Read the model definition and answer for the solid it produces. Units are mm, in the model's axes. Face numbers are marked on the shaded views. A direction names the side the tool comes from. Coordinates: 2 decimals unless noted, no trailing zeros. Write each loop counter-clockwise with the first axis right and the second up, starting at its lowest first coordinate (ties: lowest second). Pieces come first, ordered by that corner, then holes.
(1) The part is cut by section A-A, the plane z = 0. State how many separate pieces and enclosed holes the cut face has, and give its area (3 significant figures).
(2) Straight lines are drawn through the part: line 1 along X through (y, z) = (71, 12); line 2 along X through (y, z) = (11.25, 0); line 3 along Y through (x, z) = (16, 0). For each, find the intervals that lie inside material, in ascending order.
(3) Given pin 1 (8 mm diameter, centred on y = 54, z = -11, fed in from +X); pin 2 (9 mm diameter, centred on x = 13.5, y = 62, fed in from +Z); pin 3 (5.5 mm diameter, centred on y = 11, z = 18.5, fed in from -X); pin 4 (8 mm diameter, centred on x = -22, y = 39.5, fed in from -Z), each flat-ended and moving along its own axis, determine where each tip first touches the part or whether it passes through.
(4) The part is cut by section C-C, the plane x = -4. Determine the outline of the cut face in (y, z), and give its area (3 significant figures).
(5) The part is cut by section D-D, the plane y = 20. Determine the outline of the cut face in (x, z).
(6) Which of the six approach directions +Z, -Z, +X, -X, +Y, -Y give full straight-line access (tool end or side, diameter ignored) to the marked faces 4, 5 and 6?
(7) The part is cut by section B-B, the plane y = 79. Determine the outline of the cut face in (x, z).
(8) Determine the mould class of the marked faces 1, 2 and 3 for opening direction Y: pulls with the +Y half, pulls with the -Y half, needs draft (parallel to the pull), parting line crosses it, or undercut.
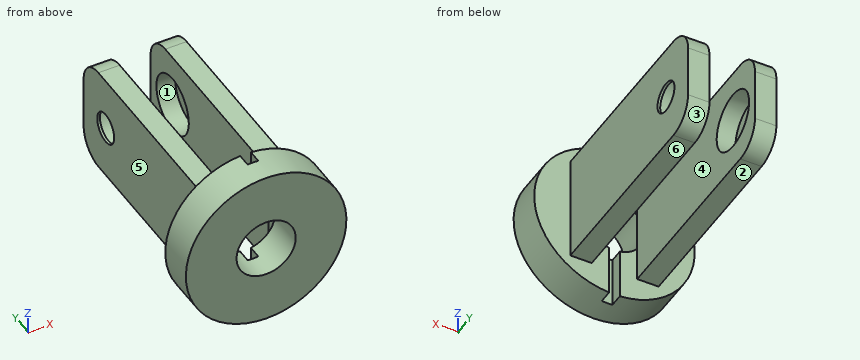
```python
from build123d import *

# Parameters (mm, degrees)
SKETCH1_R               = 30
BOSS_EXTRUDE1_DEPTH     = 14
SKETCH2_R               = 11.05
CUT_EXTRUDE1_DEPTH      = 45.676615807
SKETCH5_W               = 8
SKETCH5_H               = 40
BOSS_EXTRUDE2_DEPTH     = 80
FILLET1_R               = 10
CUT_EXTRUDE4_START      = -5
CUT_EXTRUDE4_DEPTH      = 5
CUT_EXTRUDE5_DEPTH      = 15.5
CUT_EXTRUDE5_DEPTH_BACK = 15.5
SKETCH12_R              = 11
CUT_EXTRUDE6_REACH      = 111.079
SKETCH13_R              = 5.75


with BuildPart() as part:
    # Sketch1 → Boss-Extrude1 (new body)
    with BuildSketch(Plane(origin=(0, 0, 0), x_dir=(1, 0, 0), z_dir=(0, 1, 0))):
        with Locations(Location((0, 0, 0), (0, 0, 90))):
            Circle(SKETCH1_R)
    extrude(amount=BOSS_EXTRUDE1_DEPTH)

    # Sketch2 → Cut-Extrude1 (cut, through all)
    with BuildSketch(Plane.XZ):
        with Locations(Location((0, 0, 0), (0, 0, 270))):
            Circle(SKETCH2_R)
    extrude(amount=-CUT_EXTRUDE1_DEPTH, mode=Mode.SUBTRACT)

    # Sketch5 → Boss-Extrude2 (add)
    with BuildSketch(Plane(origin=(0, 14, 0), x_dir=(1, 0, 0), z_dir=(0, 1, 0))):
        with Locations((-12.5, 0)):
            Rectangle(SKETCH5_W, SKETCH5_H)
        with Locations((12.5, 0)):
            Rectangle(SKETCH5_W, SKETCH5_H)
    extrude(amount=BOSS_EXTRUDE2_DEPTH)

    # Fillet1
    fillet1_edges = [part.edges().sort_by_distance(p)[0] for p in [
        (-12.5, 94, 20),
        (-12.5, 94, -20),
        (12.5, 94, 20),
        (12.5, 94, -20),
    ]]
    fillet(fillet1_edges, radius=FILLET1_R)

    # Sketch8 → Cut-Extrude4 (cut)
    with BuildSketch(Plane(origin=(0, 14, 0), x_dir=(1, 0, 0), z_dir=(0, 1, 0)).offset(CUT_EXTRUDE4_START)):
        with BuildLine():
            Line((2, 29.933259094), (2, -29.933259094))
            ThreePointArc((2, -29.933259094), (0, -30), (-2, -29.933259094))
            Line((-2, -29.933259094), (-2, 29.933259094))
            ThreePointArc((-2, 29.933259094), (0, 30), (2, 29.933259094))
        make_face()
    extrude(amount=CUT_EXTRUDE4_DEPTH, mode=Mode.SUBTRACT)

    # Sketch12 → Cut-Extrude5 (cut, two sides: drawn at the far end of the back side and taken through both)
    with BuildSketch(Plane(origin=(0, 0, 0), x_dir=(0, 0, -1), z_dir=(1, 0, 0)).offset(-CUT_EXTRUDE5_DEPTH_BACK)):
        with Locations((0, 79)):
            Circle(SKETCH12_R)
    extrude(amount=CUT_EXTRUDE5_DEPTH + CUT_EXTRUDE5_DEPTH_BACK, mode=Mode.SUBTRACT)

    # Cut-Extrude6: up to this face of the body (flat: up to its plane)
    cut_extrude6_end = Plane(part.part.faces().sort_by_distance((16.5, 53.48656843, 0))[0])
    # Sketch13 → Cut-Extrude6 (cut, up to the picked face)
    with BuildSketch(Plane.ZY.offset(16.5), mode=Mode.PRIVATE) as cut_extrude6_sk1:
        with Locations((0, 79)):
            Circle(SKETCH13_R)
    cut_extrude6_tool1 = split(extrude(cut_extrude6_sk1.sketch, amount=-CUT_EXTRUDE6_REACH, mode=Mode.PRIVATE), bisect_by=cut_extrude6_end, keep=Keep.BOTH, mode=Mode.PRIVATE)
    add(cut_extrude6_tool1.solids().sort_by(Axis((-16.5, 79, 0), (1, 0, 0)))[0], mode=Mode.SUBTRACT)


solid = part.part
```
Computed:
1. separate pieces: 4
1. enclosed holes: 0
1. area: 1,480 mm2
2. line 1: x = -16.5 to -8.5, 8.5 to 16.5
2. line 2: x = -30 to -11.05, 11.05 to 30
2. line 3: y = 0 to 73.25, 84.75 to 94
3. pin 1: stops at x = 16.5
3. pin 2: stops at z = 20
3. pin 3: stops at x = -25.53
3. pin 4: passes through
4. outline: (0, -29.73) - (14, -29.73) - (14, -10.3) - (0, -10.3) - close; (0, 10.3) - (14, 10.3) - (14, 29.73) - (0, 29.73) - close
4. area: 544 mm2
5. outline: (-16.5, -20) - (-8.5, -20) - (-8.5, 20) - (-16.5, 20) - close; (8.5, -20) - (16.5, -20) - (16.5, 20) - (8.5, 20) - close
6. face 4: +Z, -Z, +Y
6. face 5: +Z, -Z, -X, +Y
6. face 6: -Z, +X, -X, +Y
7. outline: (-16.5, -20) - (-8.5, -20) - (-8.5, -11) - (-15.5, -11) - (-15.5, -5.75) - (-16.5, -5.75) - close; (-16.5, 5.75) - (-15.5, 5.75) - (-15.5, 11) - (-8.5, 11) - (-8.5, 20) - (-16.5, 20) - close; (8.5, -20) - (16.5, -20) - (16.5, -5.75) - (15.5, -5.75) - (15.5, -11) - (8.5, -11) - close; (8.5, 11) - (15.5, 11) - (15.5, 5.75) - (16.5, 5.75) - (16.5, 20) - (8.5, 20) - close
8. face 1: undercut
8. face 2: needs draft
8. face 3: pulls with the +Y half
